For this review, use the dimensioned drawing (mm, ordinates from the lowest corner) and the shaded views. A direction names the side the tool comes from. Round coordinates to 2 decimals unless told otherwise and drop trailing zeros. Loops run counter-clockwise (first coordinate to the right, second up) from the corner with the lowest first, then second, coordinate; pieces in that order, holes last. Notation, with made-up numbers: (16.25, 49.5) -> (46.25, 49.5) arc R20 ccw to (46.25, 65.5) -> close; hole circle Ø11 at (70.5, -35.75). An arc over 180 degrees is marked (long way). Use one line per item in the form item = value. Start each with the question number.
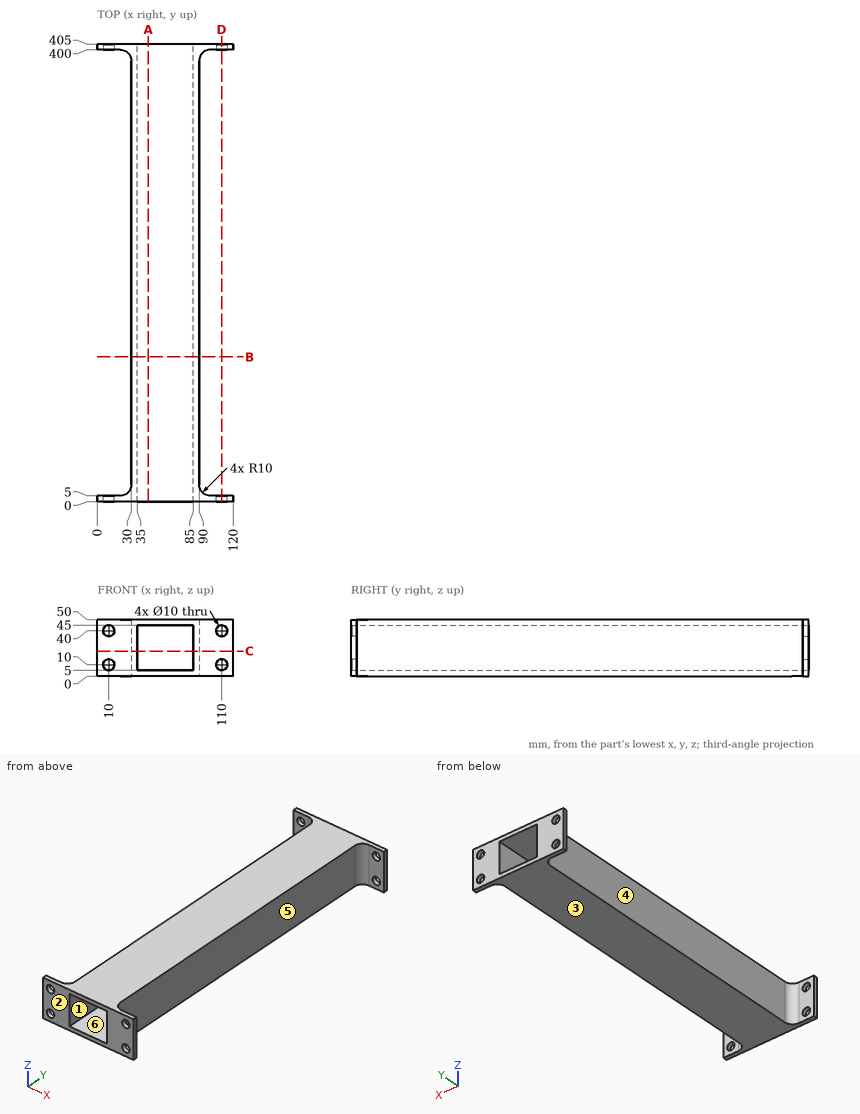
Item 1: Take a section at C-C on z = 22. Give the boundary of the cut face in (x, y), plus the area to 3 significant figures.
Item 2: Wall thickness on line 1 (X direction, y = 403.15, z = 40); line 2 (Z direction, x = 110, y = 3.3); line 3 (X direction, y = 251.5, z = 29): over which ranges is each line inside the solid? List them lowest first.
Item 3: Take a section at B-B on y = 128. Give the boundary of the cut face in (x, z), plus the area to 3 significant figures.
Item 4: Machinability: for the marked faces 4, 5 and 6, which of the approach directions +Z, -Z, +X, -X, +Y, -Y give a long, thin tool a straight path to every point of the face, cutting with its end or side? Answer none if there is none.
Item 5: For P1, Ø8, axis at x = 57, z = 41.5, coming from the -Y side; P2, Ø12, axis at y = 152, z = 30, coming from the -X side; P3, Ø12, axis at y = 138.5, z = 20.5, coming from the +X side, all flat-tipped, find the tip position at first contact; note any pin that passes through.
Item 6: Take a section at D-D on x = 110. Give the boundary of the cut face in (y, z), plus the area to 3 significant figures.
Item 7: Take a section at A-A on x = 45. Give the boundary of the cut face in (y, z).
Item 8: Draft analysis for pull direction Z (two halves, no side actions). For the marked faces 1, 2 and 3, state which applies: +Z half, -Z half, draft (parallel to the pull), parting line (faces both ways), or undercut.
Results:
q1.outline = (0, 0) -> (35, 0) -> (35, 405) -> (0, 405) -> (0, 400) -> (20, 400) arc R10 cw to (30, 390) -> (30, 15) arc R10 cw to (20, 5) -> (0, 5) -> close; (85, 0) -> (120, 0) -> (120, 5) -> (100, 5) arc R10 cw to (90, 15) -> (90, 390) arc R10 cw to (100, 400) -> (120, 400) -> (120, 405) -> (85, 405) -> close
q1.area = 4,740 mm2
q2.line_1 = 0 to 5, 15 to 35, 85 to 105, 115 to 120
q2.line_2 = 0 to 5, 15 to 35, 45 to 50
q2.line_3 = 30 to 35, 85 to 90
q3.outline = (30, 0) -> (90, 0) -> (90, 50) -> (30, 50) -> close; hole (35, 5) -> (85, 5) -> (85, 45) -> (35, 45) -> close
q3.area = 1,000 mm2
q4.face_4 = +Z, -Z, -X
q4.face_5 = +Z, -Z, +X
q4.face_6 = +Y, -Y
q5.P1 = 0
q5.P2 = 30
q5.P3 = 90
q6.outline = (0, 0) -> (5, 0) -> (5, 5) -> (0, 5) -> close; (0, 15) -> (5, 15) -> (5, 35) -> (0, 35) -> close; (0, 45) -> (5, 45) -> (5, 50) -> (0, 50) -> close; (400, 0) -> (405, 0) -> (405, 5) -> (400, 5) -> close; (400, 15) -> (405, 15) -> (405, 35) -> (400, 35) -> close; (400, 45) -> (405, 45) -> (405, 50) -> (400, 50) -> close
q6.area = 300 mm2
q7.outline = (0, 0) -> (405, 0) -> (405, 5) -> (0, 5) -> close; (0, 45) -> (405, 45) -> (405, 50) -> (0, 50) -> close
q8.face_1 = undercut
q8.face_2 = draft
q8.face_3 = -Z half
